from build123d import *

# Parameters (mm, degrees)
SKETCH1_R           = 6.35
BOSS_EXTRUDE1_DEPTH = 15.24
SKETCH3_W           = 12.7
SKETCH3_H           = 10.16
BOSS_EXTRUDE2_DEPTH = 8.89
CUT_EXTRUDE2_DEPTH  = 26.746881365
SKETCH5_R           = 1.524
BOSS_EXTRUDE3_DEPTH = 10.16


with BuildPart() as part:
    # Sketch1 → Boss-Extrude1 (new body)
    with BuildSketch(Plane(origin=(0, 0, 0), x_dir=(1, 0, 0), z_dir=(0, 1, 0))):
        with Locations(Location((0, 0, 0), (0, 0, 90))):
            Circle(SKETCH1_R)
    extrude(amount=BOSS_EXTRUDE1_DEPTH)

    # Sketch3 → Boss-Extrude2 (add)
    with BuildSketch(Plane(origin=(0, 15.24, 0), x_dir=(1, 0, 0), z_dir=(0, 1, 0))):
        Rectangle(SKETCH3_W, SKETCH3_H)
    extrude(amount=BOSS_EXTRUDE2_DEPTH)

    # Sketch4 → Cut-Extrude2 (cut, through all)
    with BuildSketch(Plane(origin=(0, 24.13, 0), x_dir=(1, 0, 0), z_dir=(0, 1, 0))):
        with BuildLine():
            ThreePointArc((3.81, 5.08), (0, 6.35), (-3.81, 5.08))
            Line((-3.81, 5.08), (3.81, 5.08))
        make_face()
        with BuildLine():
            Line((3.81, -5.08), (-3.81, -5.08))
            ThreePointArc((-3.81, -5.08), (0, -6.35), (3.81, -5.08))
        make_face()
    extrude(amount=-CUT_EXTRUDE2_DEPTH, mode=Mode.SUBTRACT)

    # Sketch5 → Boss-Extrude3 (add)
    with BuildSketch(Plane(origin=(0, 24.13, 0), x_dir=(1, 0, 0), z_dir=(0, 1, 0))):
        with Locations(Location((0, 0, 0), (0, 0, 270))):
            Circle(SKETCH5_R)
    extrude(amount=BOSS_EXTRUDE3_DEPTH)


solid = part.part
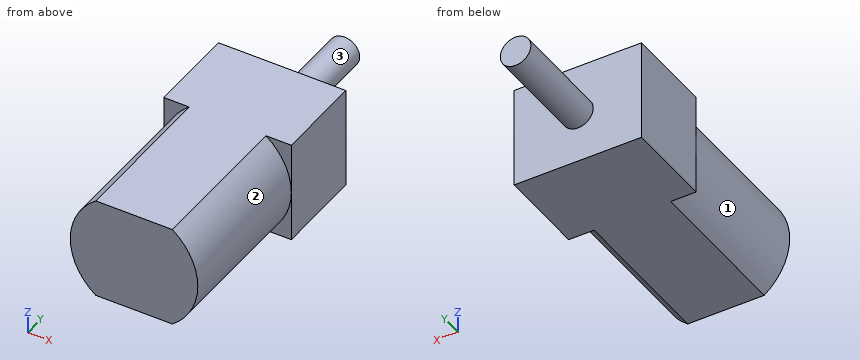
For this review, take the finished solid that the model builds, in its own axes (mm). Face numbers are marked on the shaded views. A direction names the side the tool comes from. Give positions to 0.01 mm unless a question says otherwise; leave off trailing zeros. Loops run counter-clockwise (first coordinate to the right, second up) from the corner with the lowest first, then second, coordinate; pieces in that order, holes last. Notation, with made-up numbers: (87.5, 7.25) - (99.5, 7.25) arc R18 ccw to (99.5, 22.25) - close; hole circle Ø8 at (42.5, 63). An arc over 180 degrees is marked (long way). Write each question's results on one line, items separated by ' | '.
(1) Take a section at C-C (y = 30). Give the boundary of the cut face in (x, z).
Conclusion:
outline: circle Ø3.05 at (0, 0)
(2) Take a section at D-D (z = 0.75). Give the boundary of the cut face in (x, y), then the cut area to 3 significant figures.
Conclusion:
outline: (-6.35, 15.24) - (-6.31, 15.24) - (-6.31, 0) - (6.31, 0) - (6.31, 15.24) - (6.35, 15.24) - (6.35, 24.13) - (1.33, 24.13) - (1.33, 34.29) - (-1.33, 34.29) - (-1.33, 24.13) - (-6.35, 24.13) - close | area: 332 mm^2
(3) For pin 1 Ø1.3 at (x, z) = (-5, 3) entering from -Y; pin 2 Ø2 at (x, z) = (5, 1) entering from +Y; pin 3 Ø2 at (y, z) = (27, 1) entering from +X; pin 4 Ø1.5 at (y, z) = (5, -1.5) entering from +X, all flat-tipped, find the tip position at first contact; note any pin that passes through.
Conclusion:
pin 1: y = 0 | pin 2: y = 24.13 | pin 3: x = 1.52 | pin 4: x = 6.31
(4) Take a section at A-A (x = 0). Give the boundary of the cut face in (y, z).
Conclusion:
outline: (0, -5.08) - (24.13, -5.08) - (24.13, -1.52) - (34.29, -1.52) - (34.29, 1.52) - (24.13, 1.52) - (24.13, 5.08) - (0, 5.08) - close
(5) For line 1 along Y through (x, z) = (2.75, 4.25); line 2 along Y through (x, z) = (5, -4); line 3 along Z through (x, y) = (1.25, 26), list the stretches that pass through material, from the lowest coordinate up.
Conclusion:
line 1: 0 to 24.13 | line 2: 15.24 to 24.13 | line 3: -0.87 to 0.87
(6) Take a section at B-B (z = -3). Give the boundary of the cut face in (x, y), then the cut area to 3 significant figures.
Conclusion:
outline: (-6.35, 15.24) - (-5.6, 15.24) - (-5.6, 0) - (5.6, 0) - (5.6, 15.24) - (6.35, 15.24) - (6.35, 24.13) - (-6.35, 24.13) - close | area: 283 mm^2
(7) For the marked faces 1, 2 and 3, list the 3-axis set-ups (+Z, -Z, +X, -X, +Y, -Y) from which the entire face can be reached by the end or side of a thin tool; tool diameter is ignored.
Conclusion:
face 1: -X, -Y | face 2: +X, -Y | face 3: +Y
